Part model, mm, in its own coordinate system. Face numbers are marked on the shaded views. Round coordinates to 2 decimals unless told otherwise and drop trailing zeros. Loops run counter-clockwise (first coordinate to the right, second up) from the corner with the lowest first, then second, coordinate; pieces in that order, holes last. Notation, with made-up numbers: (33, 58.25) - (90, 58.25) arc R19 cw to (90, 74.25) - close; hole circle Ø3 at (73.25, 61). An arc over 180 degrees is marked (long way). Write each question's results on one line, items separated by ' | '. Start each with the question number.
(1) Cut at B-B, the plane z = 39. List the corners of the cut face in (x, y) (3 decimals), then the cut area to 3 significant figures.
(2) Mould opens along X. For the marked faces 1 and 2 say: released by +X, released by -X, zero draft, split by the parting line, or undercut.
(3) Flat gauge pins, fed straight in: P1, Ø10, axis at x = -19, z = 0, coming from the -Y side; P2, Ø3.5, axis at x = -1, z = -54, coming from the -Y side. Where does each tip first touch, or does it go through?
(4) Cut at A-A, the plane y = -3. List the corners of the cut face in (x, z) (3 decimals).
(5) Drill centre lines: L1, parallel to Z at x = 0, y = -7.35 (3 decimals); L2, parallel to X at y = -6.5, z = -38 (3 decimals); L3, parallel to Z at x = -17, y = -6 (3 decimals). Where is each one in solid material? Low to high.
(6) Cut at C-C, the plane x = -10.5. List the corners of the cut face in (y, z) (3 decimals), then the cut area to 3 significant figures.
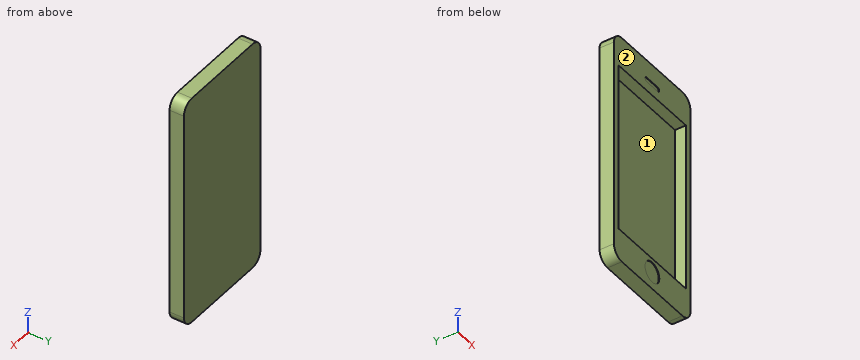
from build123d import *

# Parameters (mm, degrees)
F0_W     = 51.7
F0_H     = 90.39
F0_W_2   = 10.8
F0_H_2   = 2.3
F1_DEPTH = 7.6
F2_R     = 6.07
F3_DEPTH = 1.8
F4_R     = 1.14999
F5_DEPTH = 7.3
F6_DEPTH = 7.3


# Not quite as in the source:
# - a fillet or chamfer is up to 0.001 mm smaller than in the source, because OpenCascade refuses the exact size


with BuildPart() as f1:
    # F0 (on Front) → F1 (new body)
    with BuildSketch(Plane.XZ):
        Polygon((0, -61.915), (29.285, -61.915), (29.285, 61.915), (-29.285, 61.915), (-29.285, -61.915), align=None)
        with BuildLine():
            ThreePointArc((5.45, -52.765), (3.8537319575, -56.6187319575), (0, -58.215))
            ThreePointArc((0, -58.215), (-3.8537319575, -48.9112680425), (5.45, -52.765))
        make_face(mode=Mode.SUBTRACT)
        Rectangle(F0_W, F0_H, mode=Mode.SUBTRACT)
        with Locations((0, 51.165)):
            Rectangle(F0_W_2, F0_H_2, mode=Mode.SUBTRACT)
    extrude(amount=F1_DEPTH)

    # F2
    f2_edges = [f1.edges().sort_by_distance(p)[0] for p in [
        (-29.285, -3.8, 61.915),
        (29.285, -3.8, 61.915),
        (-29.285, -3.8, -61.915),
        (29.285, -3.8, -61.915),
    ]]
    fillet(f2_edges, radius=F2_R)

    # F0 (on Front) → F3 (join)
    with BuildSketch(Plane.XZ):
        Rectangle(F0_W, F0_H)
    extrude(amount=F3_DEPTH)

    # F4 (radius 1.15 in the source; OpenCascade refuses exactly that, so slightly less here)
    f4_edges = [f1.edges().sort_by_distance(p)[0] for p in [
        (-5.4, -3.8, 52.315),
        (5.4, -3.8, 52.315),
        (5.4, -3.8, 50.015),
        (-5.4, -3.8, 50.015),
    ]]
    fillet(f4_edges, radius=F4_R)

    # F0 (on Front) → F5 (join)
    with BuildSketch(Plane.XZ):
        with Locations((0, 51.165)):
            Rectangle(F0_W_2, F0_H_2)
    extrude(amount=F5_DEPTH)

    # F0 (on Front) → F6 (join)
    with BuildSketch(Plane.XZ):
        with BuildLine():
            ThreePointArc((5.45, -52.765), (-3.8537319575, -48.9112680425), (0, -58.215))
            ThreePointArc((0, -58.215), (3.8537319575, -56.6187319575), (5.45, -52.765))
        make_face()
    extrude(amount=F6_DEPTH)


solid = f1.part
A:
1) outline: (-29.285, -7.6) - (-25.85, -7.6) - (-25.85, -1.8) - (25.85, -1.8) - (25.85, -7.6) - (29.285, -7.6) - (29.285, 0) - (-29.285, 0) - close | area: 145 mm2
2) face 1: undercut | face 2: zero draft
3) P1: y = -1.8 | P2: y = -7.3
4) outline: (-29.285, -55.845) arc R6.07 ccw to (-23.215, -61.915) - (23.215, -61.915) arc R6.07 ccw to (29.285, -55.845) - (29.285, 55.845) arc R6.07 ccw to (23.215, 61.915) - (-23.215, 61.915) arc R6.07 ccw to (-29.285, 55.845) - close; hole (-25.85, -45.195) - (25.85, -45.195) - (25.85, 45.195) - (-25.85, 45.195) - close
5) L1: -61.915 to -58.215, -47.315 to -45.195, 45.195 to 50.015, 52.315 to 61.915 | L2: -29.285 to -25.85, 25.85 to 29.285 | L3: -61.915 to -45.195, 45.195 to 61.915
6) outline: (-7.6, -61.915) - (0, -61.915) - (0, 61.915) - (-7.6, 61.915) - (-7.6, 45.195) - (-1.8, 45.195) - (-1.8, -45.195) - (-7.6, -45.195) - close | area: 417 mm2
